Here's how the part is built. I have some questions about the finished solid (model axes, mm). A direction names the side the tool comes from. Give positions to 0.01 mm unless a question says otherwise; leave off trailing zeros. Write each loop counter-clockwise with the first axis right and the second up, starting at its lowest first coordinate (ties: lowest second). Pieces come first, ordered by that corner, then holes. Notation, with made-up numbers: (7.5, 7) - (26.5, 7) arc R9 ccw to (26.5, 12) - close; hole circle Ø5 at (85, -5.5). An arc over 180 degrees is marked (long way). Write each question's results on one line, items separated by ' | '. Start each with the question number.
Item 1: Which directions (+Z, -Z, +X, -X, +Y, -Y) give clear straight access to the entire face, cutting with the end or side of a thin tool? Please do faces 4 (the flat face through (0, 10, -162.5)), 5 (the conical face through (-52.491, 71.485, -166.684)), 6 (the flat face through (-114, 10, 96.505)), 7 (the flat face through (-1, -5, 80.255)).
Item 2: Please list where these lines run through material, in increasing order: line 1 along Z through (x, y) = (116.5, 13); line 2 along X through (y, z) = (141.45, 0); line 3 along X through (y, z) = (141, 0).
Item 3: Suppose I cut it at A-A on y = 103. List the corners of the cut face in (x, z) for me.
Item 4: We'd pull the mould along Y, two halves only. Please class faces 1 (the flat face through (112, 22, 16.505)), 2 (the flat face through (0, 50, -169)), 3 (the flat face through (-75, -10, -2)): +Y half, -Y half, draft (parallel to the pull), parting line (faces both ways), or undercut.
Item 5: Will these pins go through, and if not, where does the flat tip stop? P1, Ø1, axis at y = 41, z = -92.5, coming from the -X side; P2, Ø2, axis at x = 88, y = 65.5, coming from the -Z side; P3, Ø12, axis at x = 115, y = 32.5, coming from the -Z side; P4, Ø2.5, axis at x = 12.8, z = -152.8, coming from the -Y side.
```python
from build123d import *

# Parameters (mm, degrees)
SKETCH1_R                = 175
BOSS_EXTRUDE1_DEPTH      = 10
CUT_EXTRUDE1_DEPTH       = 248.68932153
CUT_EXTRUDE1_DEPTH_BACK  = 248.68932153
SKETCH3_W                = 35
SKETCH3_H                = 75
SKETCH3_H_2              = 35
SKETCH4_W                = 35
SKETCH4_H                = 75
CUT_EXTRUDE2_DEPTH       = 5
SKETCH5_W                = 45
SKETCH5_H                = 45
SKETCH5_W_2              = 35
SKETCH5_H_2              = 35
BOSS_EXTRUDE3_DEPTH      = 15
BOSS_EXTRUDE4_DEPTH      = 40
BOSS_EXTRUDE6_DEPTH      = 5
SKETCH9_W                = 45
SKETCH9_H                = 45
BOSS_EXTRUDE7_DEPTH      = 5
CUT_EXTRUDE14_DEPTH      = 252.545224562
CUT_EXTRUDE14_DEPTH_BACK = 252.545224562
SKETCH36_W               = 105
SKETCH36_H               = 160.510321068
SKETCH45_W               = 5
SKETCH45_H               = 24
BOSS_EXTRUDE14_DEPTH     = 25
SKETCH46_R               = 1.7
CUT_EXTRUDE18_DEPTH      = 25
SKETCH49_R               = 2
CUT_EXTRUDE20_DEPTH      = 250.299017246
SKETCH57_R               = 2
CUT_EXTRUDE24_DEPTH      = 5.5
SKETCH58_W               = 60
SKETCH58_H               = 30
CUT_EXTRUDE25_DEPTH      = 371.41362016


with BuildPart() as part:
    # Sketch1 → Boss-Extrude1 (new body)
    with BuildSketch(Plane(origin=(0, 0, 0), x_dir=(1, 0, 0), z_dir=(0, 1, 0))):
        with Locations(Location((0, 0, 0), (0, 0, 270))):
            Circle(SKETCH1_R)
    extrude(amount=-BOSS_EXTRUDE1_DEPTH)

    # Sketch3 → Cut-Extrude1 (cut, two sides: drawn at the far end of the back side and taken through both)
    with BuildSketch(Plane.XZ.offset(10).offset(-CUT_EXTRUDE1_DEPTH_BACK)):
        with Locations((-110, 59.005160534)):
            Rectangle(SKETCH3_W, SKETCH3_H)
        with Locations((110, 59.005160534)):
            Rectangle(SKETCH3_W, SKETCH3_H)
        with Locations((0, -140)):
            Rectangle(SKETCH3_W, SKETCH3_H_2)
    extrude(amount=CUT_EXTRUDE1_DEPTH + CUT_EXTRUDE1_DEPTH_BACK, mode=Mode.SUBTRACT)

    # Sketch4 → Cut-Extrude2 (cut)
    with BuildSketch(Plane(origin=(0, 0, 0), x_dir=(1, 0, 0), z_dir=(0, 1, 0))):
        Polygon((57.5, -21.505160534), (57.5, -96.505160534), (57.5, -121.505160534), (92.5, -121.505160534), (92.5, -96.505160534), (92.5, -21.505160534), align=None)
        with Locations((110, -59.005160534)):
            Rectangle(SKETCH4_W, SKETCH4_H)
        Polygon((-57.5, -21.505160534), (-92.5, -21.505160534), (-92.5, -96.505160534), (-92.5, -121.505160534), (-57.5, -121.505160534), (-57.5, -96.505160534), align=None)
    extrude(amount=-CUT_EXTRUDE2_DEPTH, mode=Mode.SUBTRACT)

    # Sketch5 → Boss-Extrude3 (add)
    with BuildSketch(Plane(origin=(0, 0, 0), x_dir=(1, 0, 0), z_dir=(0, 1, 0))):
        with Locations((0, 140)):
            Rectangle(SKETCH5_W, SKETCH5_H)
        with Locations((0, 140)):
            Rectangle(SKETCH5_W_2, SKETCH5_H_2, mode=Mode.SUBTRACT)
    extrude(amount=BOSS_EXTRUDE3_DEPTH)

    # Sketch6 → Boss-Extrude4 (add)
    with BuildSketch(Plane(origin=(0, 0, 0), x_dir=(1, 0, 0), z_dir=(0, 1, 0))):
        Polygon((127.5, -21.505160534), (92.5, -21.505160534), (92.5, -16.505160534), (132.5, -16.505160534), (132.5, -101.505160534), (110, -101.505160534), (110, -96.505160534), (127.5, -96.505160534), align=None)
        Polygon((-127.5, -21.505160534), (-127.5, -96.505160534), (-110, -96.505160534), (-110, -101.505160534), (-132.5, -101.505160534), (-132.5, -16.505160534), (-92.5, -16.505160534), (-92.5, -21.505160534), align=None)
    extrude(amount=BOSS_EXTRUDE4_DEPTH)

    # Sketch8 → Boss-Extrude6 (add)
    with BuildSketch(Plane(origin=(0, 40, 0), x_dir=(1, 0, 0), z_dir=(0, 1, 0))):
        Polygon((-97.5, -16.505160534), (-92.5, -16.505160534), (-92.5, -101.505160534), (-110, -101.505160534), (-132.5, -101.505160534), (-132.5, -16.505160534), align=None)
        Polygon((132.5, -16.505160534), (97.5, -16.505160534), (92.5, -16.505160534), (92.5, -101.505160534), (110, -101.505160534), (132.5, -101.505160534), align=None)
    extrude(amount=BOSS_EXTRUDE6_DEPTH)

    # Sketch9 → Boss-Extrude7 (add)
    with BuildSketch(Plane(origin=(0, 15, 0), x_dir=(1, 0, 0), z_dir=(0, 1, 0))):
        with Locations((0, 140)):
            Rectangle(SKETCH9_W, SKETCH9_H)
    extrude(amount=BOSS_EXTRUDE7_DEPTH)

    # Sketch36 → Cut-Extrude14 (cut, two sides: drawn at the far end of the back side and taken through both)
    with BuildSketch(Plane(origin=(0, 0, 0), x_dir=(1, 0, 0), z_dir=(0, 1, 0)).offset(-CUT_EXTRUDE14_DEPTH_BACK)):
        Rectangle(SKETCH36_W, SKETCH36_H)
    extrude(amount=CUT_EXTRUDE14_DEPTH + CUT_EXTRUDE14_DEPTH_BACK, mode=Mode.SUBTRACT)

    # Sketch45 → Boss-Extrude14 (add)
    with BuildSketch(Plane(origin=(0, -5, 0), x_dir=(1, 0, 0), z_dir=(0, 1, 0))):
        with Locations((71.2, -76.505160534)):
            Rectangle(SKETCH45_W, SKETCH45_H)
        with Locations((-71.2, -76.505160534)):
            Rectangle(SKETCH45_W, SKETCH45_H)
    extrude(amount=BOSS_EXTRUDE14_DEPTH)

    # Sketch46 → Cut-Extrude18 (cut)
    with BuildSketch(Plane.ZY.offset(-68.7)):
        with Locations((79.505160534, -2.2)):
            Circle(SKETCH46_R)
        with Locations(Location((79.505160534, 14.8, 0), (0, 0, 180))):
            Circle(SKETCH46_R)
        with BuildLine():
            Line((68.005160534, 7.5), (68.105160534, 7.5))
            ThreePointArc((68.105160534, 7.5), (70.005160534, 5.6), (71.905160534, 7.5))
            Line((71.905160534, 7.5), (72.005160534, 7.5))
            ThreePointArc((72.005160534, 7.5), (70.005160534, 9.5), (68.005160534, 7.5))
        make_face()
    cut_extrude18 = extrude(amount=-CUT_EXTRUDE18_DEPTH, mode=Mode.SUBTRACT)

    # Mirror1: Cut-Extrude18 across plane
    add(cut_extrude18.mirror(Plane.ZY), mode=Mode.SUBTRACT)

    # Sketch49 → Cut-Extrude20 (cut, through all)
    with BuildSketch(Plane(origin=(0, 20, 0), x_dir=(1, 0, 0), z_dir=(0, 1, 0))):
        with BuildLine():
            ThreePointArc((-10.803300859, 152.803300859), (-12.037933994, 154.651059924), (-14.217514421, 154.217514421))
            Line((-14.217514421, 154.217514421), (-12.803300859, 152.803300859))
            Line((-12.803300859, 152.803300859), (-11.389087297, 151.389087297))
            ThreePointArc((-11.389087297, 151.389087297), (-10.955541794, 152.037933994), (-10.803300859, 152.803300859))
        make_face()
        with BuildLine():
            Line((-12.803300859, 152.803300859), (-14.217514421, 154.217514421))
            ThreePointArc((-14.217514421, 154.217514421), (-14.217514421, 151.389087297), (-11.389087297, 151.389087297))
            Line((-11.389087297, 151.389087297), (-12.803300859, 152.803300859))
        make_face()
        with Locations(Location((12.803300859, 152.803300859, 0), (0, 0, 270))):
            Circle(SKETCH49_R)
        with Locations(Location((-12.803300859, 127.196699141, 0), (0, 0, 270))):
            Circle(SKETCH49_R)
        with Locations(Location((12.803300859, 127.196699141, 0), (0, 0, 270))):
            Circle(SKETCH49_R)
    extrude(amount=-CUT_EXTRUDE20_DEPTH, mode=Mode.SUBTRACT)

    # Sketch51 → Revolve1 (revolve)
    with BuildSketch(Plane.XY, mode=Mode.PRIVATE) as revolve1_sk:
        Polygon((-160, 145), (-174.5, 145), (-175, 0), (-170, 0), align=None)
    revolve(revolve1_sk.sketch.rotate(Axis((0, 0, 0), (0, 1, 0)), 270), axis=Axis((0, 0, 0), (0, 1, 0)))

    # Sketch57 → Cut-Extrude24 (cut)
    with BuildSketch(Plane(origin=(0, 145, 0), x_dir=(1, 0, 0), z_dir=(0, 1, 0))):
        with Locations(Location((170, 0, 0), (0, 0, 270))):
            Circle(SKETCH57_R)
        with Locations(Location((-170, 0, 0), (0, 0, 90))):
            Circle(SKETCH57_R)
        with Locations(Location((0, 170, 0), (0, 0, 270))):
            Circle(SKETCH57_R)
        with Locations(Location((0, -170, 0), (0, 0, 90))):
            Circle(SKETCH57_R)
    extrude(amount=-CUT_EXTRUDE24_DEPTH, mode=Mode.SUBTRACT)

    # Sketch58 → Cut-Extrude25 (cut, through all)
    with BuildSketch(Plane.XY.offset(-117.5)):
        with Locations((0, 65)):
            Rectangle(SKETCH58_W, SKETCH58_H)
    extrude(amount=-CUT_EXTRUDE25_DEPTH, mode=Mode.SUBTRACT)


solid = part.part
```
Checked values:
1) face 4: none | face 5: +Y | face 6: -Y | face 7: +Y, -Y
2) line 1: z = -130.53 to -122.57, 16.51 to 21.51, 96.51 to 101.51, 122.57 to 130.53 | line 2: x = -174.51 to -172, -168 to -160.24, 160.24 to 168, 172 to 174.51 | line 3: x = -174.51 to -172, -168 to -160.28, 160.28 to 168, 172 to 174.51
3) outline: circle Ø349.29 at (0, 0); hole circle Ø325.79 at (0, 0)
4) face 1: draft | face 2: undercut | face 3: -Y half
5) P1: stops at x = -148.7 | P2: stops at z = -151.58 | P3: stops at z = -136.77 | P4: passes through
